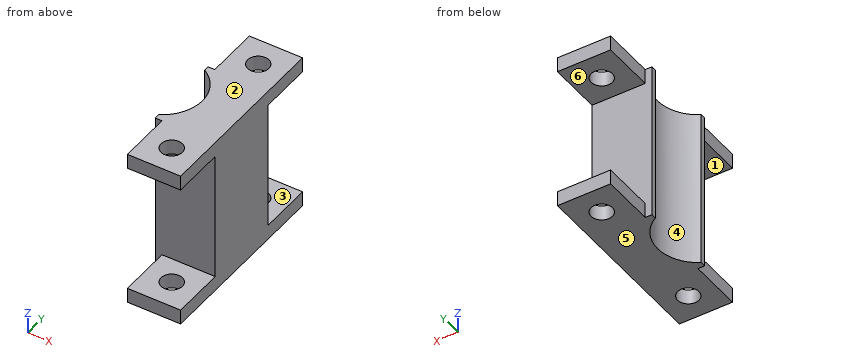
```python
from build123d import *

# Parameters (mm, degrees)
SKETCH_R          = 1.6
PAD_DEPTH         = 12
SKETCH001_W       = 8
SKETCH001_H       = 32
POCKET_DEPTH      = 12.001
POCKET_DEPTH_BACK = 12.001
SKETCH002_W       = 24
SKETCH002_H       = 16
POCKET001_DEPTH   = 9.75


with BuildPart() as part:
    # Sketch → Pad (new body, symmetric)
    with BuildSketch(Plane.XY):
        with BuildLine():
            ThreePointArc((-6.1, -6.1), (0, 0), (-6.1, 6.1))
            Line((-6.1, 6.1), (-2.1, 6.1))
            Line((-2.1, 6.1), (-2.1, 14.1))
            Line((-2.1, 14.1), (5.9, 14.1))
            Line((5.9, 14.1), (5.9, -14.1))
            Line((-2.1, -14.1), (5.9, -14.1))
            Line((-2.1, -6.1), (-2.1, -14.1))
            Line((-6.1, -6.1), (-2.1, -6.1))
        make_face()
        with Locations((1.9, 10)):
            Circle(SKETCH_R, mode=Mode.SUBTRACT)
        with Locations((1.9, -10)):
            Circle(SKETCH_R, mode=Mode.SUBTRACT)
    extrude(amount=PAD_DEPTH, both=True)

    # Sketch001 → Pocket (cut, two sides)
    with BuildSketch(Plane.XY) as pocket_sk:
        with Locations((-7.1, 0)):
            Rectangle(SKETCH001_W, SKETCH001_H)
    extrude(amount=-POCKET_DEPTH, mode=Mode.SUBTRACT)
    extrude(pocket_sk.sketch, amount=POCKET_DEPTH_BACK, mode=Mode.SUBTRACT)

    # Sketch002 → Pocket001 (cut, symmetric)
    with BuildSketch(Plane.XY):
        with Locations((5.9, 14.1)):
            Rectangle(SKETCH002_W, SKETCH002_H)
        with Locations((5.9, -14.1)):
            Rectangle(SKETCH002_W, SKETCH002_H)
    extrude(amount=POCKET001_DEPTH, both=True, mode=Mode.SUBTRACT)


solid = part.part
```
Read the model definition and answer for the solid it produces. Units are mm, in the model's axes. Face numbers are marked on the shaded views. A direction names the side the tool comes from. Give positions to 0.01 mm unless a question says otherwise; leave off trailing zeros. Write each loop counter-clockwise with the first axis right and the second up, starting at its lowest first coordinate (ties: lowest second). Pieces come first, ordered by that corner, then holes. Notation, with made-up numbers: M -7.75,55.5 L 36.25,55.5 A22 cw 36.25,65.5 Z; hole C -4.75,39.5 d8. An arc over 180 degrees is marked long. Put each result on its own line as item: value. Start each with the question number.
1. Each of these flat-tipped pins is pushed along its axis until it touches: pin 1 Ø4.5 at (x, z) = (1.5, 4) entering from -Y; pin 2 Ø2.5 at (y, z) = (-11.5, -11) entering from -X; pin 3 Ø1 at (y, z) = (3.5, -0.5) entering from -X; pin 4 Ø1.5 at (x, y) = (-2, 4) entering from +Z. Where does it stop, or does it pass through?
2. Which of the six approach directions +Z, -Z, +X, -X, +Y, -Y give full straight-line access (tool end or side, diameter ignored) to the marked faces 1 and 2?
3. The part is cut by section A-A, the plane x = 1.9. Give the vertices of the cut face in (y, z).
4. The part is cut by section C-C, the plane z = -1.5. Give the vertices of the cut face in (x, y).
5. The part is cut by section B-B, the plane y = -10. Give the vertices of the cut face in (x, z), and give its area (3 significant figures).
6. For a pull along Z with two mould halves and no side action, classify the marked faces 3, 4, 5 and 6 as released by +Z, released by -Z, zero draft, split by the parting line, or undercut.
7. The part is cut by section D-D, the plane x = 5.5. Give the vertices of the cut face in (y, z).
8. Consider line 1 along Y through (x, z) = (1.9, 10.5); line 2 along Z through (x, y) = (5.5, -11.75); line 3 along X through (y, z) = (-10, 11.45). Determine where each line is inside the solid, lowest interval first.
Final values:
1. pin 1: stops at y = -6.1
1. pin 2: stops at x = -2.1
1. pin 3: stops at x = -1.49
1. pin 4: stops at z = 12
2. face 1: +X, -X, -Y
2. face 2: +Z, +X, -X, +Y, -Y
3. outline: M -14.1,-12 L -11.6,-12 L -11.6,-9.75 L -14.1,-9.75 Z; M -14.1,9.75 L -11.6,9.75 L -11.6,12 L -14.1,12 Z; M -8.4,-12 L 8.4,-12 L 8.4,-9.75 L 6.1,-9.75 L 6.1,9.75 L 8.4,9.75 L 8.4,12 L -8.4,12 L -8.4,9.75 L -6.1,9.75 L -6.1,-9.75 L -8.4,-9.75 Z; M 11.6,-12 L 14.1,-12 L 14.1,-9.75 L 11.6,-9.75 Z; M 11.6,9.75 L 14.1,9.75 L 14.1,12 L 11.6,12 Z
4. outline: M -3.1,-6.1 L 5.9,-6.1 L 5.9,6.1 L -3.1,6.1 L -3.1,5.31 A6.1 cw -3.1,-5.31 Z
5. outline: M -2.1,-12 L 0.3,-12 L 0.3,-9.75 L -2.1,-9.75 Z; M -2.1,9.75 L 0.3,9.75 L 0.3,12 L -2.1,12 Z; M 3.5,-12 L 5.9,-12 L 5.9,-9.75 L 3.5,-9.75 Z; M 3.5,9.75 L 5.9,9.75 L 5.9,12 L 3.5,12 Z
5. area: 21.6 mm²
6. face 3: undercut
6. face 4: zero draft
6. face 5: released by -Z
6. face 6: undercut
7. outline: M -14.1,-12 L 14.1,-12 L 14.1,-9.75 L 6.1,-9.75 L 6.1,9.75 L 14.1,9.75 L 14.1,12 L -14.1,12 L -14.1,9.75 L -6.1,9.75 L -6.1,-9.75 L -14.1,-9.75 Z
8. line 1: y = -14.1 to -11.6, -8.4 to 8.4, 11.6 to 14.1
8. line 2: z = -12 to -9.75, 9.75 to 12
8. line 3: x = -2.1 to 0.3, 3.5 to 5.9
